```python
from build123d import *

# Parameters (mm, degrees)
SKETCH1_W            = 16
SKETCH1_H            = 8
BOSS_EXTRUDE1_DEPTH  = 9.6
SKETCH2_R            = 2.4
BOSS_EXTRUDE2_DEPTH  = 1.6
LPATTERN1_COUNT      = 2
LPATTERN1_PITCH      = 8
LPATTERN1_COUNT_DIR2 = 4
LPATTERN1_PITCH_DIR2 = 8
SHELL1_T             = -1.6


with BuildPart() as part:
    # Sketch1 → Boss-Extrude1 (new body)
    with BuildSketch(Plane(origin=(0, 0, 0), x_dir=(1, 0, 0), z_dir=(0, 1, 0))):
        with Locations((8, 4)):
            Rectangle(SKETCH1_W, SKETCH1_H)
    extrude(amount=BOSS_EXTRUDE1_DEPTH)

    # Sketch2 → Boss-Extrude2 (add)
    with BuildSketch(Plane(origin=(0, 9.6, 0), x_dir=(1, 0, 0), z_dir=(0, 1, 0))):
        with Locations(Location((12, 4, 0), (0, 0, 90))):
            Circle(SKETCH2_R)
    boss_extrude2 = extrude(amount=BOSS_EXTRUDE2_DEPTH)

    # LPattern1: Boss-Extrude2 2 × 4, 6 skipped
    with Locations(*[(-i * LPATTERN1_PITCH, 0, -j * LPATTERN1_PITCH_DIR2) for i in range(LPATTERN1_COUNT) for j in range(LPATTERN1_COUNT_DIR2) if (i, j) not in ((0, 0), (0, 1), (0, 2), (0, 3), (1, 1), (1, 2), (1, 3))]):
        add(boss_extrude2)

    # Shell1
    shell1_openings = [part.faces().sort_by_distance(p)[0] for p in [
        (8, 0, -4),
    ]]
    offset(amount=SHELL1_T, openings=shell1_openings, kind=Kind.INTERSECTION)


solid = part.part
```
Check sheet for the modelled part. Datum: model origin and axes. Units: mm. A direction names the side the tool comes from. Give positions to 0.01 mm unless a question says otherwise; leave off trailing zeros. Loops run counter-clockwise (first coordinate to the right, second up) from the corner with the lowest first, then second, coordinate; pieces in that order, holes last. Notation, with made-up numbers: M -5.75,25 L 22.25,25 A30 cw 22.25,47 Z; hole C 47.25,81.25 d5. An arc over 180 degrees is marked long. Answer in a Markdown table with one row per item.
1) Thickness scan on line 1 (X direction, y = 8.75, z = -4); line 2 (X direction, y = 1.25, z = -3.75); line 3 (Z direction, x = 2.25, y = 7). Record the ranges inside material, lowest first.
Solutions:
| item | result |
|---|---|
| line 1 | x = 0 to 3.2, 4.8 to 11.2, 12.8 to 16 |
| line 2 | x = 0 to 1.6, 14.4 to 16 |
| line 3 | z = -8 to -6.4, -1.6 to 0 |
2) Cross-section at D-D (z = -5.25). Enter the section's corners in (x, y), plus the area to 3 significant figures.
Solutions:
| item | result |
|---|---|
| outline | M 0,0 L 1.6,0 L 1.6,8 L 14.4,8 L 14.4,0 L 16,0 L 16,9.6 L 14.05,9.6 L 14.05,11.2 L 9.95,11.2 L 9.95,9.6 L 6.05,9.6 L 6.05,11.2 L 1.95,11.2 L 1.95,9.6 L 0,9.6 Z |
| area | 64.3 mm^2 |
3) Cross-section at C-C (x = 12). Enter the section's corners in (y, z).
Solutions:
| item | result |
|---|---|
| outline | M 0,-8 L 9.6,-8 L 9.6,-6.4 L 11.2,-6.4 L 11.2,-1.6 L 9.6,-1.6 L 9.6,0 L 0,0 L 0,-1.6 L 8,-1.6 L 8,-3.2 L 9.6,-3.2 L 9.6,-4.8 L 8,-4.8 L 8,-6.4 L 0,-6.4 Z |
4) Mould release check, pull along X, two halves, no side actions. Record for faces 1 (the face through (16, 5, -4)), 2 (the face through (4, 11.2, -4)), 3 (the face through (3.28, 10.39, -6.29)): released by +X, released by -X, zero draft, split by the parting line, or undercut.
Solutions:
| item | result |
|---|---|
| face 1 | released by +X |
| face 2 | zero draft |
| face 3 | undercut |
5) Cross-section at B-B (y = 8.25). Enter the section's corners in (x, z).
Solutions:
| item | result |
|---|---|
| outline | M 0,-8 L 16,-8 L 16,0 L 0,0 Z; hole C 4,-4 d1.6; hole C 12,-4 d1.6 |
6) Tool access check on faces 4 (the face through (14.4, 4, -4)), 5 (the face through (12, 11.2, -4)), 6 (the face through (9.976, 10.389, -5.29)). Record the directions out of +Z, -Z, +X, -X, +Y, -Y that give a thin tool (end or side, any length) a straight path to the whole face; none if there is none.
Solutions:
| item | result |
|---|---|
| face 4 | -Y |
| face 5 | +Z, -Z, +X, -X, +Y |
| face 6 | +Y |
7) Cross-section at A-A (y = 4.5). Enter the section's corners in (x, z).
Solutions:
| item | result |
|---|---|
| outline | M 0,-8 L 16,-8 L 16,0 L 0,0 Z; hole M 1.6,-6.4 L 14.4,-6.4 L 14.4,-1.6 L 1.6,-1.6 Z |
8) Depth check by flat-ended pin: pin 1 (1.8 mm diameter, centred on x = 4, z = -4.5, fed in from -Y); pin 2 (0.5 mm diameter, centred on x = 12, z = -4, fed in from -Y). Enter the tip coordinate at first touch or a pass-through.
Solutions:
| item | result |
|---|---|
| pin 1 | stops at y = 8 |
| pin 2 | stops at y = 9.6 |
